Read the model definition and answer for the solid it produces. Units are mm, in the model's axes. A direction names the side the tool comes from. Coordinates: 2 decimals unless noted, no trailing zeros. Loops run counter-clockwise (first coordinate to the right, second up) from the corner with the lowest first, then second, coordinate; pieces in that order, holes last. Notation, with made-up numbers: (64.5, 65.5) -> (72.5, 65.5) arc R20 ccw to (72.5, 104.5) -> close; hole circle Ø3 at (-36.75, -32). An arc over 180 degrees is marked (long way). Answer as a JSON object with one key per item and string values. Group by question number.
1) Section B-B, the plane z = 5.5 is taken. Give the vertices of the cut face in (x, y).
2) Section C-C, the plane x = -1.5 is taken. Give the vertices of the cut face in (y, z), plus the area to 3 significant figures.
3) Consider probe 1 along Z at (x, y) = (-8.75, 3); probe 2 along X at (y, z) = (-0.25, 5); probe 3 along X at (y, z) = (-3.75, -0.75). Determine where each line is inside the solid, lowest interval first. Write a range as [from, to].
4) Section D-D, the plane y = 3.75 is taken. Give the vertices of the cut face in (x, z).
5) Determine the mould class of faces 5 (the face through (-6, 0, 8)), 6 (the face through (-8, 0, 3)) for opening direction X: released by +X, released by -X, zero draft, split by the parting line, or undercut.
6) Flat-ended cylindrical pins translate along their axes: P1, Ø3, axis at x = 8, y = -3, coming from the -Z side; P2, Ø3, axis at x = 3.5, z = 6, coming from the -Y side; P3, Ø5, axis at x = -2, z = 5.5, coming from the -Y side. Find the tip coordinate at first contact, or state that the pin passes through.
7) Which of the six approach directions +Z, -Z, +X, -X, +Y, -Y give full straight-line access (tool end or side, diameter ignored) to faces 1 (the face through (0, 0, 7)), 2 (the face through (-0.06, 2.25, -0.49)), 3 (the face through (0, 0, -1)), 4 (the face through (0, 0, 6))?
Autodesk Inventor part; units mm, degrees
ref_plane "Work Plane1" through (0, 0, 3) normal (0, 0, 1) x (1, 0, 0)
ref_plane "Work Plane2" through (0, -8.7656, 3) normal (0, 0, 1) x (1, 0, 0)
ref_plane "YZ Plane" through (0, 0, 0) normal (1, 0, 0) x (0, 1, 0)
sketch "Sketch1" plane through (0, 0, 0) normal (0, 0, 1) x (1, 0, 0)
  arc A0 (-3.7827, 3.4604) -> (-3.7827, -3.4604) centre (-6.25, 0) ccw
  arc A1 (-3.7827, 3.4604) -> (3.7827, 3.4604) centre (0, 8.7656) ccw
  arc A2 (3.7827, -3.4604) -> (-3.7827, -3.4604) centre (0, -8.7656) ccw
  arc A3 (3.7827, -3.4604) -> (3.7827, 3.4604) centre (6.25, 0) ccw
  line L0 (0, 0) -> (0, 4.5286) construction
  circle A4 centre (-6.25, 0) radius 1.75
  circle A5 centre (6.25, 0) radius 1.75
  point P0 (0, 2.25)
  point P1 (0, -2.25)
  dimension "d0" = 4.5
  dimension "d2" = 8.5
  dimension "d4" = 8.5
  dimension "d5" = 12.5
  dimension "d6" = 3.5
  dimension "d7" = 3.5
extrude "Extrusion1" add sketch "Sketch1" against normal blind 1
extrude "Extrusion2" add sketch "Sketch1" against normal blind 2 contours A4 | A5
extrude "Extrusion3" add sketch "Sketch1" along normal blind 6 contours A4 | A5
ref_plane "Work Plane1" through (0, 0, 3) normal (0, 0, 1) x (1, 0, 0)
mirror "Mirror1" about plane through (0, 0, 3) normal (0, 0, 1) of "Extrusion1", "Extrusion2"
ref_plane "Work Plane2" through (0, -8.7656, 3) normal (0, 0, 1) x (1, 0, 0)
equation "\"d4\" = d2"
equation "\"d7\" = d6"
properties part number "Outer Chain"
Determined:
{
 "1": {"outline": "circle Ø3.5 at (-6.25, 0); circle Ø3.5 at (6.25, 0)"},
 "2": {"outline": "(-2.42, -1) -> (2.42, -1) -> (2.42, 0) -> (-2.42, 0) -> close; (-2.42, 6) -> (2.42, 6) -> (2.42, 7) -> (-2.42, 7) -> close", "area": "9.70 mm²"},
 "3": {"probe 1": "[-1, 0], [6, 7]", "probe 2": "[-7.98, -4.52], [4.52, 7.98]", "probe 3": "[-8.25, -4.25], [4.25, 8.25]"},
 "4": {"outline": "(-8.25, -1) -> (-4.25, -1) -> (-4.25, 0) -> (-8.25, 0) -> close; (-8.25, 6) -> (-4.25, 6) -> (-4.25, 7) -> (-8.25, 7) -> close; (4.25, -1) -> (8.25, -1) -> (8.25, 0) -> (4.25, 0) -> close; (4.25, 6) -> (8.25, 6) -> (8.25, 7) -> (4.25, 7) -> close"},
 "5": {"face 5": "zero draft", "face 6": "undercut"},
 "6": {"P1": "z = -1", "P2": "y = -4.06", "P3": "y = -3.85"},
 "7": {"face 1": "+Z", "face 2": "+Z, -Z, +Y", "face 3": "-Z", "face 4": "none"}
}
